Geometry: see drawing. Coordinates: mm, zero at the bounding-box minimum. A direction names the side the tool comes from. Round coordinates to 2 decimals unless told otherwise and drop trailing zeros. Write each loop counter-clockwise with the first axis right and the second up, starting at its lowest first coordinate (ties: lowest second). Pieces come first, ordered by that corner, then holes. Notation, with made-up numbers: M -10,10.25 L 28,10.25 A21 cw 28,22.25 Z; hole C 43,55 d5. An arc over 180 degrees is marked long. Use one line per item in the form item = value. Start each with the question number.
Item 1: Section query C-C (y = 19.5). Return loops of the section in (x, z).
Item 2: Section query B-B (x = 57.5). Return loops of the section in (y, z) (1 decimal), and give its area (3 significant figures).
Item 3: Section query D-D (x = 17). Return loops of the section in (y, z), and give its area (3 significant figures).
Item 4: Reachability of the marked faces 1 and 2 from +Z, -Z, +X, -X, +Y, -Y: full face, straight path, thin tool, end or side. Return the list, or none.
Item 5: Pin query (flat end, axial travel): pin 1 Ø12.5 at (y, z) = (16.5, 47) entering from +X; pin 2 Ø12.5 at (x, y) = (56.5, 7.5) entering from +Z. Return the tip coordinate at first contact, or that it passes through.
Item 6: Pull-direction query (X, two-part tool) for the marked faces 3, 4 and 5; classes: pulls with the +X half, pulls with the -X half, needs draft (parallel to the pull), parting line crosses it, or undercut.
Item 7: Ray query, probe 1 along Z at (x, y) = (40, 5); probe 2 along X at (y, z) = (14.5, 47); probe 3 along X at (y, z) = (7.5, 7) (1 decimal). Return the intervals inside material, ascending.
Item 8: Section query A-A (y = 6). Return loops of the section in (x, z) (1 decimal), and give its area (3 significant figures).
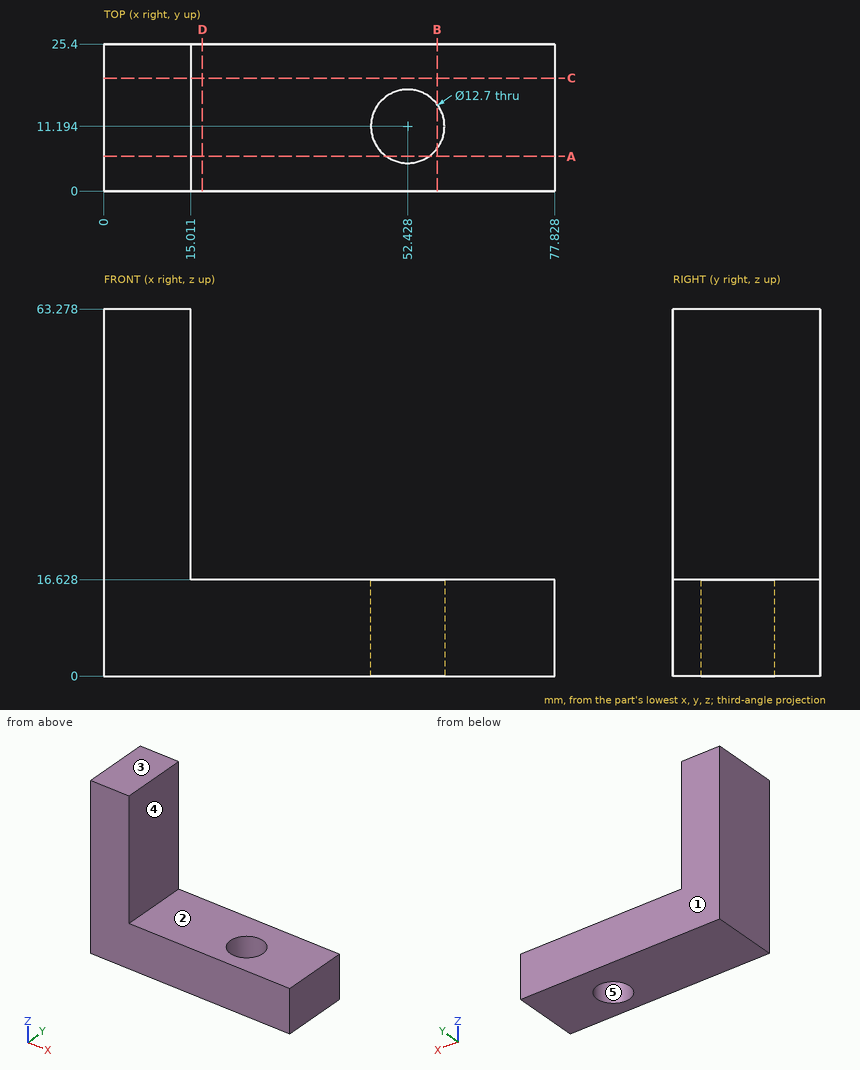
Working result:
q1.outline = M 0,0 L 77.83,0 L 77.83,16.63 L 15.01,16.63 L 15.01,63.28 L 0,63.28 Z
q2.outline = M 0,0 L 7.4,0 L 7.4,16.6 L 0,16.6 Z; M 15,0 L 25.4,0 L 25.4,16.6 L 15,16.6 Z
q2.area = 295 mm²
q3.outline = M 0,0 L 25.4,0 L 25.4,16.63 L 0,16.63 Z
q3.area = 422 mm²
q4.face_1 = +Z, -Z, +X, -X, +Y
q4.face_2 = +Z, +X, +Y, -Y
q5.pin_1 = 15.01
q5.pin_2 = 16.63
q6.face_3 = needs draft
q6.face_4 = pulls with the +X half
q6.face_5 = undercut
q7.probe_1 = 0 to 16.63
q7.probe_2 = 0 to 15.01
q7.probe_3 = 0 to 47.3, 57.6 to 77.8
q8.outline = M 0,0 L 48.8,0 L 48.8,16.6 L 15,16.6 L 15,63.3 L 0,63.3 Z; M 56.1,0 L 77.8,0 L 77.8,16.6 L 56.1,16.6 Z
q8.area = 1,870 mm²
